Source: CAD feature listing. Evaluate the final solid. Frame: model axes, mm. A direction names the side the tool comes from. Round coordinates to 2 decimals unless told otherwise and drop trailing zeros. Loops run counter-clockwise (first coordinate to the right, second up) from the corner with the lowest first, then second, coordinate; pieces in that order, holes last.
Item 1: Access query for faces 1 (the flat face through (-8, 2, 26)), 2 (the flat face through (-1, 15, 26)). Directions: +Z, -Z, +X, -X, +Y, -Y. A direction counts if a zero-diameter tool reaches every point of the face in a straight line with its end or side. Return the directions, or none.
Item 2: First-contact query: P1, Ø2.5, axis at y = 9, z = 42, coming from the -X side; P2, Ø2, axis at y = 10.5, z = 46.5, coming from the -X side. Flat tips, straight axial feed; report the tip coordinate or a pass-through.
Item 3: Pull-direction query (Y, two-part tool) for faces 3 (the flat face through (-15, 1, 26)), 4 (the flat face through (-8, 0, 26)), 5 (the cylindrical face through (-1.014, 10.352, 40.526)); classes: released by +Y, released by -Y, zero draft, split by the parting line, or undercut.
Item 4: Section query D-D on z = 34. Return loops of the section in (x, y).
Item 5: Section query C-C on x = -12. Return loops of the section in (y, z).
Item 6: Section query A-A on z = 42. Return loops of the section in (x, y).
Item 7: Ray query, L1, parallel to Y at x = -0.5, z = 42; L2, parallel to Y at x = -3.25, z = 37; L3, parallel to X at y = 10, z = 31.5. Return the intervals inside material, ascending.
Item 8: Section query B-B on y = 9. Return loops of the section in (x, z), then the cut area to 3 significant figures.
```python
from build123d import *

# Parameters (mm, degrees)
EXTRUDE_1_DEPTH     = 52
FILLET_1_R          = 0.8
SKETCH_3_R          = 2
CUT_EXTRUDE_2_DEPTH = 2


with BuildPart() as part:
    # 草图1 → 凸台-拉伸1 (new body)
    with BuildSketch(Plane.XY):
        Polygon((0, 0), (0, 15), (-2, 15), (-2, 2), (-15, 2), (-15, 0), align=None)
    extrude(amount=EXTRUDE_1_DEPTH)

    # 圆角1
    fillet_1_edges = [part.edges().sort_by_distance(p)[0] for p in [
        (-15, 2, 26),
        (-2, 15, 26),
    ]]
    fillet(fillet_1_edges, radius=FILLET_1_R)

    # 草图3 → 切除-拉伸2 (cut)
    with BuildSketch(Plane.ZY.offset(2)):
        with Locations((42, 9)):
            Circle(SKETCH_3_R)
    extrude(amount=-CUT_EXTRUDE_2_DEPTH, mode=Mode.SUBTRACT)


solid = part.part
```
Data:
1. face 1: +Z, -Z, -X, +Y
1. face 2: +Z, -Z, +X, -X, +Y
2. P1: passes through
2. P2: stops at x = -2
3. face 3: zero draft
3. face 4: released by -Y
3. face 5: undercut
4. outline: (-15, 0) - (0, 0) - (0, 15) - (-1.2, 15) arc R0.8 ccw to (-2, 14.2) - (-2, 2) - (-14.2, 2) arc R0.8 ccw to (-15, 1.2) - close
5. outline: (0, 0) - (2, 0) - (2, 52) - (0, 52) - close
6. outline: (-15, 0) - (0, 0) - (0, 7) - (-2, 7) - (-2, 2) - (-14.2, 2) arc R0.8 ccw to (-15, 1.2) - close; (-2, 11) - (0, 11) - (0, 15) - (-1.2, 15) arc R0.8 ccw to (-2, 14.2) - close
7. L1: y = 0 to 7, 11 to 15
7. L2: y = 0 to 2
7. L3: x = -2 to 0
8. outline: (-2, 0) - (0, 0) - (0, 40) - (-2, 40) - close; (-2, 44) - (0, 44) - (0, 52) - (-2, 52) - close
8. area: 96.0 mm2
